Part model, mm, in its own coordinate system. Face numbers are marked on the shaded views. A direction names the side the tool comes from. Give positions to 0.01 mm unless a question says otherwise; leave off trailing zeros. Order: outer loops, then holes, each group sorted by start corner. A loop starts at its lowest first (then second) coordinate and runs counter-clockwise, first axis right, second up. Notation, with made-up numbers: (22.25, 50.5) -> (37.25, 50.5) arc R23 cw to (37.25, 61.5) -> close; hole circle Ø4 at (-35, -3). An arc over 180 degrees is marked (long way). Write item = value, one per line. Start each with the question number.
(1) Saw through at D-D, the plane x = -7.5. List the corners of the cut face in (y, z), then the cut area to 3 significant figures.
(2) Flat gauge pins, fed straight in: pin 1 (1.5 mm diameter, centred on x = -6.5, y = -5, fed in from +Z); pin 2 (4 mm diameter, centred on y = -5, z = 5, fed in from -X). Where does each tip first touch, or does it go through?
(3) Saw through at A-A, the plane x = 0. List the corners of the cut face in (y, z).
(4) Saw through at C-C, the plane y = 7.25. List the corners of the cut face in (x, z).
(5) Which spindle directions (+Z, -Z, +X, -X, +Y, -Y) get a long thin tool onto all of the face, cutting with end or side? Do the marked faces 1 and 2. Say none if no direction does.
(6) Probe line 1 along Y through (x, z) = (-4, 11.5); line 2 along X through (y, z) = (-1, 4.5); line 3 along Y through (x, z) = (1, 18). List the from-to ranges inside material, lowest first. Write a range as from..to.
(7) Saw through at B-B, the plane z = 1.75. List the corners of the cut face in (x, y).
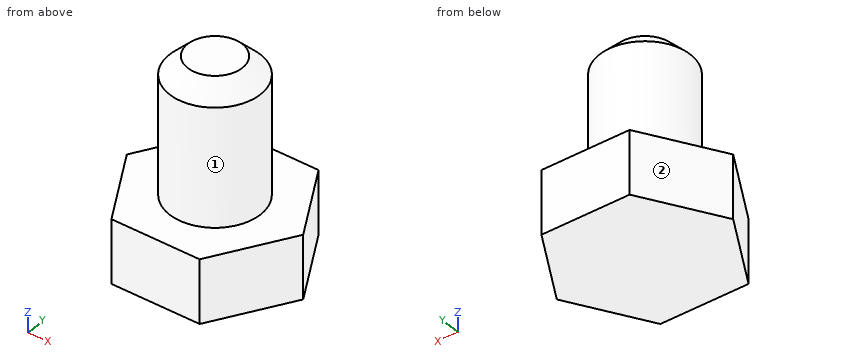
from build123d import *

# Parameters (mm, degrees)
F1_DEPTH = 7
F2_R     = 5
F3_DEPTH = 15
F4_SIZE  = 2


with BuildPart() as f1:
    # F0 (on Top) → F1 (new body)
    with BuildSketch(Plane.XY):
        Polygon((-4.907477, -8.5), (4.907477, -8.5), (9.814955, 0), (4.907477, 8.5), (-4.907477, 8.5), (-9.814955, 0), align=None)
    extrude(amount=F1_DEPTH)

    # F2 (on face) → F3 (join)
    with BuildSketch(Plane.XY.offset(7)):
        Circle(F2_R)
    extrude(amount=F3_DEPTH)

    # F4
    f4_edges = [f1.edges().sort_by_distance(p)[0] for p in [
        (-5, 0, 22),
    ]]
    chamfer(f4_edges, length=F4_SIZE)


solid = f1.part
Results list:
q1.outline = (-4.01, 0) -> (4.01, 0) -> (4.01, 7) -> (-4.01, 7) -> close
q1.area = 56.1 mm^2
q2.pin_1 = 7
q2.pin_2 = -8.08
q3.outline = (-8.5, 0) -> (8.5, 0) -> (8.5, 7) -> (5, 7) -> (5, 20) -> (3, 22) -> (-3, 22) -> (-5, 20) -> (-5, 7) -> (-8.5, 7) -> close
q4.outline = (-5.63, 0) -> (5.63, 0) -> (5.63, 7) -> (-5.63, 7) -> close
q5.face_1 = +Z
q5.face_2 = +Z, -Z, -X, +Y
q6.line_1 = -3..3
q6.line_2 = -9.24..9.24
q6.line_3 = -4.9..4.9
q7.outline = (-9.81, 0) -> (-4.91, -8.5) -> (4.91, -8.5) -> (9.81, 0) -> (4.91, 8.5) -> (-4.91, 8.5) -> close
